Print and shaded views of the part. All mm, measured from the part's lowest x, y and z. A direction names the side the tool comes from. Round coordinates to 2 decimals unless told otherwise and drop trailing zeros. Order: outer loops, then holes, each group sorted by start corner. A loop starts at its lowest first (then second) coordinate and runs counter-clockwise, first axis right, second up. Notation, with made-up numbers: (-14.5, 43.25) - (-0.5, 43.25) arc R25 cw to (-0.5, 60.25) - close; hole circle Ø6 at (19, 58). An arc over 180 degrees is marked (long way). Return JSON: item names as keys, results as strings. Group by question number.
Item 1: Saw through at D-D on z = 21.25. List the corners of the cut face in (x, y).
Item 2: Saw through at B-B on z = 13.5. List the corners of the cut face in (x, y).
Item 3: Tool access for the marked faces 1, 2 and 3: list every direction of +Z, -Z, +X, -X, +Y, -Y with a clear straight run to the whole face (end or side of a thin tool).
Item 4: Saw through at C-C on y = 2.75. List the corners of the cut face in (x, z) (1 decimal).
Item 5: Two-plate mould, pull along Z, no slides. Class the marked faces 4, 5, 6 and 7: released by +Z, released by -Z, zero draft, split by the parting line, or undercut.
Item 6: Saw through at A-A on x = 24. List the corners of the cut face in (y, z).
Item 7: Drop flat-ended pins along their axis: pin 1 (3 mm diameter, centred on y = 4, z = 6, fed in from +X) (1 decimal); pin 2 (6.5 mm diameter, centred on x = 6, z = 13.5, fed in from +Y); pin 3 (3 mm diameter, centred on x = 6, y = 6.5, fed in from -Z); pin 4 (5 mm diameter, centred on x = 27, z = 22.5, fed in from +Y). Give the stop position or say it passes through.
Item 8: Probe probe 1 along X at (y, z) = (2.75, 13.5); probe 2 along X at (y, z) = (6, 13.5); probe 3 along X at (y, z) = (10, 13.5). List the from-to ranges inside material, lowest first.
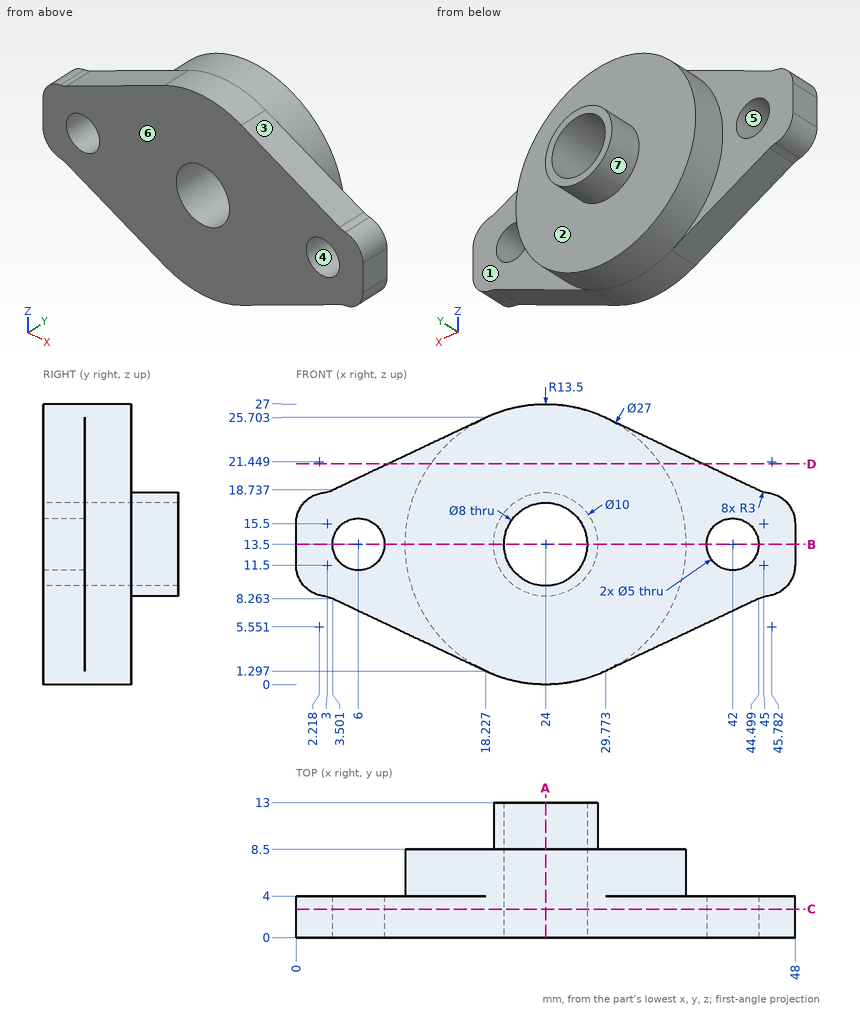
Filled in:
{
 "1": {"outline": "(8.81, 0) - (39.19, 0) - (39.19, 4) - (35.05, 4) - (35.05, 8.5) - (12.95, 8.5) - (12.95, 4) - (8.81, 4) - close"},
 "2": {"outline": "(0, 0) - (3.5, 0) - (3.5, 4) - (0, 4) - close; (8.5, 0) - (20, 0) - (20, 13) - (19, 13) - (19, 8.5) - (10.5, 8.5) - (10.5, 4) - (8.5, 4) - close; (28, 0) - (39.5, 0) - (39.5, 4) - (37.5, 4) - (37.5, 8.5) - (29, 8.5) - (29, 13) - (28, 13) - close; (44.5, 0) - (48, 0) - (48, 4) - (44.5, 4) - close"},
 "3": {"face 1": "+X, +Y", "face 2": "+Y", "face 3": "+Z, +X, +Y, -Y"},
 "4": {"outline": "(0, 11.5) arc R3 ccw to (2.6, 8.5) arc R3 cw to (3.5, 8.3) - (18.2, 1.3) arc R13.5 ccw to (29.8, 1.3) - (44.5, 8.3) arc R3 cw to (45.4, 8.5) arc R3 ccw to (48, 11.5) - (48, 15.5) arc R3 ccw to (45.4, 18.5) arc R3 cw to (44.5, 18.7) - (29.8, 25.7) arc R13.5 ccw to (18.2, 25.7) - (3.5, 18.7) arc R3 cw to (2.6, 18.5) arc R3 ccw to (0, 15.5) - close; hole circle Ø5 at (6, 13.5); hole circle Ø8 at (24, 13.5); hole circle Ø5 at (42, 13.5)"},
 "5": {"face 4": "undercut", "face 5": "undercut", "face 6": "zero draft", "face 7": "split by the parting line"},
 "6": {"outline": "(0, 0) - (8.5, 0) - (8.5, 8.5) - (13, 8.5) - (13, 9.5) - (0, 9.5) - close; (0, 17.5) - (13, 17.5) - (13, 18.5) - (8.5, 18.5) - (8.5, 27) - (0, 27) - close"},
 "7": {"pin 1": "stops at x = 42.9", "pin 2": "stops at y = 4", "pin 3": "passes through", "pin 4": "stops at y = 8.5"},
 "8": {"probe 1": "x = 0 to 3.5, 8.5 to 20, 28 to 39.5, 44.5 to 48", "probe 2": "x = 10.5 to 20, 28 to 37.5", "probe 3": "x = 19 to 20, 28 to 29"}
}
